Autodesk Inventor part; units mm, degrees
ref_plane "YZ Plane" through (0, 0, 0) normal (1, 0, 0) x (0, 1, 0)
ref_plane "XZ Plane" through (0, 0, 0) normal (0, 1, 0) x (-1, 0, 0)
ref_plane "XY Plane" through (0, 0, 0) normal (0, 0, 1) x (1, 0, 0)
sketch "Sketch1" plane through (0, 0, 0) normal (0, 1, 0) x (-1, 0, 0)
  line L0 (69.85, 69.85) -> (-69.85, 69.85)
  line L1 (-69.85, 69.85) -> (-69.85, -69.85)
  line L2 (-69.85, -69.85) -> (69.85, -69.85)
  line L3 (69.85, -69.85) -> (69.85, 69.85)
  line L4 (97.79, 0) -> (-97.79, 0)
  line L5 (0, -97.79) -> (0, 97.79)
  point P0 (0, 0)
  dimension "d0" = 139.7
  dimension "d1" = 139.7
extrude "Extrusion1" add sketch "Sketch1" along normal blind 3.175
sketch "Sketch2" plane through (0, 3.175, 0) normal (0, 1, 0) x (1, 0, 0)
  line L0 (-69.85, 69.85) -> (-69.85, -69.85)
  line L1 (-69.85, -69.85) -> (-69.85, -53.975)
  line L2 (-69.85, -53.975) -> (-53.975, -53.975)
  point P0 (0, 0)
  dimension "d4" = 15.875
  dimension "d5" = 15.875
hole "Hole1" at (-53.975, 3.175, 53.975) direction (0, -1, 0) diameter 5.5118 depth 14.1986 tip angle 118
mirror "Mirror4" about plane through (0, 0, 0) normal (0, 0, 1) of "Hole1"
mirror "Mirror5" about plane through (0, 0, 0) normal (1, 0, 0) of "Hole1", "Mirror4"
sketch "Sketch5" plane through (0, 3.175, 0) normal (0, 1, 0) x (1, 0, 0)
  point P0 (0, 0)
  point P1 (0, 0)
hole "Hole3" at (0, 3.175, 0) direction (0, -1, 0) diameter 5.5118 end through all
pattern_linear "Rectangular Pattern2" count 5 spacing 25.4 along (1, 0, 0) of "Hole3" first direction both ways yes
pattern_linear "Rectangular Pattern3" count 5 spacing 25.4 along (0, 0, 1) of "Hole3" first direction both ways yes
equation "\"d0\" = d1"
equation "\"d4\" = d5"
properties part number "DIFF_HOUSING_TOP"
Can you work these out from the model? Positions are in its coordinate system, mm. Round coordinates to 2 decimals unless told otherwise and drop trailing zeros. Loops run counter-clockwise (first coordinate to the right, second up) from the corner with the lowest first, then second, coordinate; pieces in that order, holes last. Notation, with made-up numbers: (54, 43.25) -> (94, 43.25) arc R25 cw to (94, 81.25) -> close; hole circle Ø4 at (51, 5.25). An arc over 180 degrees is marked (long way). One line per item, written item: value. Start each with the question number.
1. If I drill on probe 1 along Z at (x, y) = (54, 2.3); probe 2 along Z at (x, y) = (0, 1.6), over which ranges is the centre line in solid material (lowest first)?
2. For pin 1 (6.5 mm diameter, centred on x = 25.4, z = 0, fed in from +Y) (3 decimals); pin 2 (4.5 mm diameter, centred on x = 0, z = -50.8, fed in from +Y), each with a flat end and sliding along its axis, tell me the tip position at first contact or that it passes through.
3. If we section it at D-D, the plane z = 26: Write out the boundary of the cut face in (x, y) (3 decimals).
4. If we section it at C-C, the plane x = 25.4: Write out the boundary of the cut face in (y, z) (3 decimals).
5. If we section it at A-A, the plane x = 0: Write out the boundary of the cut face in (y, z) (3 decimals).
6. If we section it at B-B, the plane z = 0: Write out the boundary of the cut face in (x, y) (3 decimals).
7. If we mould it in two halves opening along X, with no side actions, what happens to faces 1 (the flat face through (1, 2, -69.85)), 2 (the flat face through (-69.85, 2, -1)), 3 (the flat face through (69.85, 2, 1)), 4 (the cylindrical face through (-22.955, 1.565, 1.272))? For each: pulls with the +X half, pulls with the -X half, needs draft (parallel to the pull), parting line crosses it, or undercut.
Calculated:
1. probe 1: z = -69.85 to -56.73, -51.22 to 51.22, 56.73 to 69.85
1. probe 2: z = -69.85 to -53.56, -48.04 to -28.16, -22.64 to -2.76, 2.76 to 22.64, 28.16 to 48.04, 53.56 to 69.85
2. pin 1: stops at y = 3.175
2. pin 2: passes through
3. outline: (-69.85, 0) -> (-2.69, 0) -> (-2.69, 3.175) -> (-69.85, 3.175) -> close; (2.69, 0) -> (69.85, 0) -> (69.85, 3.175) -> (2.69, 3.175) -> close
4. outline: (0, -69.85) -> (3.175, -69.85) -> (3.175, -2.756) -> (0, -2.756) -> close; (0, 2.756) -> (3.175, 2.756) -> (3.175, 69.85) -> (0, 69.85) -> close
5. outline: (0, -69.85) -> (3.175, -69.85) -> (3.175, -53.556) -> (0, -53.556) -> close; (0, -48.044) -> (3.175, -48.044) -> (3.175, -28.156) -> (0, -28.156) -> close; (0, -22.644) -> (3.175, -22.644) -> (3.175, -2.756) -> (0, -2.756) -> close; (0, 2.756) -> (3.175, 2.756) -> (3.175, 22.644) -> (0, 22.644) -> close; (0, 28.156) -> (3.175, 28.156) -> (3.175, 48.044) -> (0, 48.044) -> close; (0, 53.556) -> (3.175, 53.556) -> (3.175, 69.85) -> (0, 69.85) -> close
6. outline: (-69.85, 0) -> (-53.556, 0) -> (-53.556, 3.175) -> (-69.85, 3.175) -> close; (-48.044, 0) -> (-28.156, 0) -> (-28.156, 3.175) -> (-48.044, 3.175) -> close; (-22.644, 0) -> (-2.756, 0) -> (-2.756, 3.175) -> (-22.644, 3.175) -> close; (2.756, 0) -> (22.644, 0) -> (22.644, 3.175) -> (2.756, 3.175) -> close; (28.156, 0) -> (48.044, 0) -> (48.044, 3.175) -> (28.156, 3.175) -> close; (53.556, 0) -> (69.85, 0) -> (69.85, 3.175) -> (53.556, 3.175) -> close
7. face 1: needs draft
7. face 2: pulls with the -X half
7. face 3: pulls with the +X half
7. face 4: undercut
